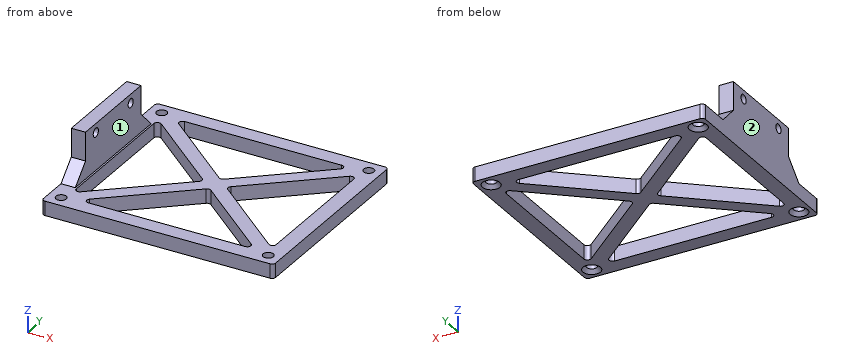
from build123d import *

# Parameters (mm, degrees)
SKETCH_W        = 65
SKETCH_H        = 56
SKETCH_R        = 1.45
PAD_DEPTH       = 4
SKETCH002_R     = 1.25
POCKET_DEPTH    = 5
SKETCH003_W     = 4
SKETCH003_H     = 27
PAD001_DEPTH    = 13
SKETCH004_R     = 1.25
POCKET001_DEPTH = 65.001
CHAMFER_SIZE    = 5
FILLET_R        = 1
CHAMFER001_SIZE = 1


with BuildPart() as part:
    # Sketch → Pad (new body)
    with BuildSketch(Plane.XY):
        with Locations((32.5, 28)):
            Rectangle(SKETCH_W, SKETCH_H)
        with Locations((3.5, 52.5)):
            Circle(SKETCH_R, mode=Mode.SUBTRACT)
        with Locations((61.5, 52.5)):
            Circle(SKETCH_R, mode=Mode.SUBTRACT)
        with Locations((3.5, 3.5)):
            Circle(SKETCH_R, mode=Mode.SUBTRACT)
        with Locations((61.5, 3.5)):
            Circle(SKETCH_R, mode=Mode.SUBTRACT)
        Polygon((7.782759, 51.5), (57.217241, 51.5), (32.5, 30.618193), align=None, mode=Mode.SUBTRACT)
        Polygon((60.5, 49.036979), (60.5, 6.963021), (35.599086, 28), align=None, mode=Mode.SUBTRACT)
        Polygon((57.217241, 4.5), (7.782759, 4.5), (32.5, 25.381807), align=None, mode=Mode.SUBTRACT)
        Polygon((4.5, 6.963021), (4.5, 49.036979), (29.400914, 28), align=None, mode=Mode.SUBTRACT)
    extrude(amount=PAD_DEPTH)

    # Sketch002 → Pocket (cut)
    with BuildSketch(Plane(origin=(-1.55844, 1.844684, 0), x_dir=(-0.763886, -0.645352, 0), z_dir=(-0.645352, 0.763886, 0))):
        with Locations((-21.5, 5.25)):
            Circle(SKETCH002_R)
        with Locations((-4.5, 5.25)):
            Circle(SKETCH002_R)
    extrude(amount=-POCKET_DEPTH, mode=Mode.SUBTRACT)

    # Sketch003 (on Face22 of Pocket) → Pad001 (join)
    with BuildSketch(Plane.XY.offset(4)):
        with Locations((2, 28)):
            Rectangle(SKETCH003_W, SKETCH003_H)
    extrude(amount=PAD001_DEPTH)

    # Sketch004 (on Face7 of Pad001) → Pocket001 (cut, through all)
    with BuildSketch(Plane(origin=(0, 0, 0), x_dir=(0, -1, 0), z_dir=(-1, 0, 0))):
        with Locations((-36.5, 14.5)):
            Circle(SKETCH004_R)
        with Locations((-19.5, 14.5)):
            Circle(SKETCH004_R)
    extrude(amount=-POCKET001_DEPTH, mode=Mode.SUBTRACT)

    # Chamfer
    chamfer_edges = [part.edges().sort_by_distance(p)[0] for p in [
        (2, 41.5, 4),
        (2, 14.5, 4),
    ]]
    chamfer(chamfer_edges, length=CHAMFER_SIZE)

    # Fillet
    fillet_edges = [part.edges().sort_by_distance(p)[0] for p in [
        (7.782759, 51.5, 2),
        (35.599086, 28, 2),
        (60.5, 6.963021, 2),
        (4.5, 6.963021, 2),
        (29.400914, 28, 2),
        (7.782759, 4.5, 2),
        (57.217241, 4.5, 2),
        (57.217241, 51.5, 2),
        (4.5, 49.036979, 2),
        (4.95, 52.5, 2),
        (32.5, 25.381807, 2),
        (32.5, 30.618193, 2),
        (60.5, 49.036979, 2),
        (0, 56, 2),
        (65, 56, 2),
        (65, 0, 2),
        (0, 0, 2),
    ]]
    fillet(fillet_edges, radius=FILLET_R)

    # Chamfer001
    chamfer001_edges = [part.edges().sort_by_distance(p)[0] for p in [
        (2.05, 52.5, 0),
        (2.05, 3.5, 0),
        (60.05, 3.5, 0),
        (60.05, 52.5, 0),
    ]]
    chamfer(chamfer001_edges, length=CHAMFER001_SIZE)


solid = part.part
Part model, mm, in its own coordinate system. Face numbers are marked on the shaded views. A direction names the side the tool comes from. Give positions to 0.01 mm unless a question says otherwise; leave off trailing zeros. Write each loop counter-clockwise with the first axis right and the second up, starting at its lowest first coordinate (ties: lowest second). Pieces come first, ordered by that corner, then holes.
1) Cut at A-A on x = 61.5. Write the cut outline in (y, z).
Resolved:
outline: (0, 0) - (1.05, 0) - (2.05, 1) - (2.05, 4) - (0, 4) - close; (4.95, 1) - (5.95, 0) - (50.05, 0) - (51.05, 1) - (51.05, 4) - (4.95, 4) - close; (53.95, 1) - (54.95, 0) - (56, 0) - (56, 4) - (53.95, 4) - close
2) Cut at D-D on y = 36.5. Write the cut outline in (x, z), then the cut area to 3 significant figures.
Resolved:
outline: (0, 0) - (4.5, 0) - (4.5, 4) - (4, 4) - (4, 13.25) - (0, 13.25) - close; (0, 15.75) - (4, 15.75) - (4, 17) - (0, 17) - close; (19.34, 0) - (25.54, 0) - (25.54, 4) - (19.34, 4) - close; (39.46, 0) - (45.66, 0) - (45.66, 4) - (39.46, 4) - close; (60.5, 0) - (65, 0) - (65, 4) - (60.5, 4) - close
area: 128 mm2
3) Which spindle directions (+Z, -Z, +X, -X, +Y, -Y) get a long thin tool onto all of the face, cutting with end or side? Do the marked faces 1 and 2. Say none if no direction does.
Resolved:
face 1: +Z, +X, +Y, -Y
face 2: +Z, -Z, -X, +Y, -Y
4) Probe L1, parallel to Y at x = 61.5, z = 3.25; L2, parallel to Z at x = 0.8, y = 19.5; L3, parallel to Y at x = 48.5, z = 3.5. List the from-to ranges inside material, lowest first.
Resolved:
L1: y = 0 to 2.05, 4.95 to 51.05, 53.95 to 56
L2: z = 0 to 13.25, 15.75 to 17
L3: y = 0 to 4.5, 11.86 to 17.1, 38.9 to 44.14, 51.5 to 56
5) Cut at C-C on x = 38.5. Write the cut outline in (y, z).
Resolved:
outline: (0, 0) - (4.5, 0) - (4.5, 4) - (0, 4) - close; (20.31, 0) - (25.55, 0) - (25.55, 4) - (20.31, 4) - close; (30.45, 0) - (35.69, 0) - (35.69, 4) - (30.45, 4) - close; (51.5, 0) - (56, 0) - (56, 4) - (51.5, 4) - close
6) Pin check, flat tips, straight feed: pin 1 (4 mm diameter, centred on y = 36.5, z = 14.5, fed in from -X); pin 2 (4 mm diameter, centred on y = 19.5, z = 14.5, fed in from +X); pin 3 (4 mm diameter, centred on x = 61.5, y = 3.5, fed in from -Z); pin 4 (4.5 mm diameter, centred on x = 1.5, z = 13, fed in from +Y). Stop position of each tip, or through.
Resolved:
pin 1: stops at x = 0
pin 2: stops at x = 4
pin 3: stops at z = 0.45
pin 4: stops at y = 41.5
7) Cut at B-B on y = 52.5. Write the cut outline in (x, z), then the cut area to 3 significant figures.
Resolved:
outline: (0, 0) - (1.05, 0) - (2.05, 1) - (2.05, 4) - (0, 4) - close; (4.95, 1) - (5.95, 0) - (59.05, 0) - (60.05, 1) - (60.05, 4) - (4.95, 4) - close; (62.95, 1) - (63.95, 0) - (65, 0) - (65, 4) - (62.95, 4) - close
area: 235 mm2
